```python
from build123d import *

# Parameters (mm, degrees)
BOSS_EXTRUDE1_DEPTH                                 = 10
SKETCH2_W                                           = 22.52
SKETCH2_H                                           = 12.02
CUT_EXTRUDE1_DEPTH                                  = 154.297097168
CBORE_FOR_00_BINDING_HEAD_MACHINE_SCREW_D           = 1.397
CBORE_FOR_00_BINDING_HEAD_MACHINE_SCREW_CBORE_D     = 3.175
CBORE_FOR_00_BINDING_HEAD_MACHINE_SCREW_CBORE_DEPTH = 0.7112


with BuildPart() as part:
    # Sketch1 → Boss-Extrude1 (new body)
    with BuildSketch(Plane.XY):
        with BuildLine():
            Line((10, 0), (140, 0))
            ThreePointArc((140, 0), (147.071067812, 2.928932188), (150, 10))
            Line((150, 10), (150, 20))
            ThreePointArc((150, 20), (147.071067812, 27.071067812), (140, 30))
            Line((140, 30), (10, 30))
            ThreePointArc((10, 30), (2.928932188, 27.071067812), (0, 20))
            Line((0, 20), (0, 10))
            ThreePointArc((0, 10), (2.928932188, 2.928932188), (10, 0))
        make_face()
    extrude(amount=BOSS_EXTRUDE1_DEPTH)

    # Sketch2 → Cut-Extrude1 (cut, through all)
    with BuildSketch(Plane(origin=(0, 0, 0), x_dir=(-1, 0, 0), z_dir=(0, 0, -1))):
        with Locations((-130.892658662, 15.006569468)):
            Rectangle(SKETCH2_W, SKETCH2_H)
    extrude(amount=-CUT_EXTRUDE1_DEPTH, mode=Mode.SUBTRACT)

    # CBORE for #00 Binding Head Machine Screw3 (through all)
    with Locations(Plane(origin=(0, 0, 0), x_dir=(-1, 0, 0), z_dir=(0, 0, -1))):
        with Locations((-146.209359197, 15.668360935), (-115.743972015, 15.453815955)):
            CounterBoreHole(CBORE_FOR_00_BINDING_HEAD_MACHINE_SCREW_D / 2, CBORE_FOR_00_BINDING_HEAD_MACHINE_SCREW_CBORE_D / 2, CBORE_FOR_00_BINDING_HEAD_MACHINE_SCREW_CBORE_DEPTH)


solid = part.part
```
Source: CAD feature listing. Evaluate the final solid. Frame: model axes, mm. A direction names the side the tool comes from. Round coordinates to 2 decimals unless told otherwise and drop trailing zeros. Loops run counter-clockwise (first coordinate to the right, second up) from the corner with the lowest first, then second, coordinate; pieces in that order, holes last.
(1) Contact query for flat-ended pins moving along their axis: pin 1 Ø5 at (x, y) = (42.5, 5.5) entering from -Z; pin 2 Ø1.5 at (y, z) = (4, 6) entering from +X; pin 3 Ø1 at (y, z) = (22.5, 3) entering from +X. Output: stop coordinate, or through.
From the geometry:
pin 1: stops at z = 0
pin 2: stops at x = 148.51
pin 3: stops at x = 149.8
(2) Material intervals for probe 1 along Y at (x, z) = (123.5, 1.75); probe 2 along X at (y, z) = (15.25, 5.25); probe 3 along X at (y, z) = (14.5, 9), sorted ascending.
From the geometry:
probe 1: y = 0 to 9, 21.02 to 30
probe 2: x = 0 to 115.08, 116.41 to 119.63, 142.15 to 145.65, 146.77 to 150
probe 3: x = 0 to 119.63, 142.15 to 150
(3) Access query for faces 5 (the flat face through (142.153, 15, 5)), 6 (the flat face through (147, 16, 0.711)), 7 (the cylindrical face through (147.15, 26.99, 4.93)). Directions: +Z, -Z, +X, -X, +Y, -Y. A direction counts if a zero-diameter tool reaches every point of the face in a straight line with its end or side. Return the directions, or none.
From the geometry:
face 5: +Z, -Z
face 6: -Z
face 7: +Z, -Z, +X, +Y
(4) Section query A-A (y = 11.25). Output: boundary loops of the cut face in (x, z).
From the geometry:
outline: (0, 0) - (119.63, 0) - (119.63, 10) - (0, 10) - close; (142.15, 0) - (150, 0) - (150, 10) - (142.15, 10) - close
(5) Section query D-D (y = 26). Output: boundary loops of the cut face in (x, z).
From the geometry:
outline: (2, 0) - (148, 0) - (148, 10) - (2, 10) - close
(6) Section query B-B (x = 132). Output: boundary loops of the cut face in (y, z), and give its area (3 significant figures).
From the geometry:
outline: (0, 0) - (9, 0) - (9, 10) - (0, 10) - close; (21.02, 0) - (30, 0) - (30, 10) - (21.02, 10) - close
area: 180 mm2
(7) Section query C-C (z = 7.5). Output: boundary loops of the cut face in (x, y).
From the geometry:
outline: (0, 10) arc R10 ccw to (10, 0) - (140, 0) arc R10 ccw to (150, 10) - (150, 20) arc R10 ccw to (140, 30) - (10, 30) arc R10 ccw to (0, 20) - close; hole circle Ø1.4 at (115.74, 15.45); hole (119.63, 9) - (142.15, 9) - (142.15, 21.02) - (119.63, 21.02) - close; hole circle Ø1.4 at (146.21, 15.67)
(8) Pull-direction query (X, two-part tool) for faces 1 (the flat face through (115, 15, 0.711)), 2 (the flat face through (119.633, 15, 5)), 3 (the flat face through (150, 15, 5)), 4 (the cylindrical face through (3.01, 27.15, 4.93)); classes: +X half, -X half, draft (parallel to the pull), parting line (faces both ways), or undercut.
From the geometry:
face 1: undercut
face 2: undercut
face 3: +X half
face 4: -X half
